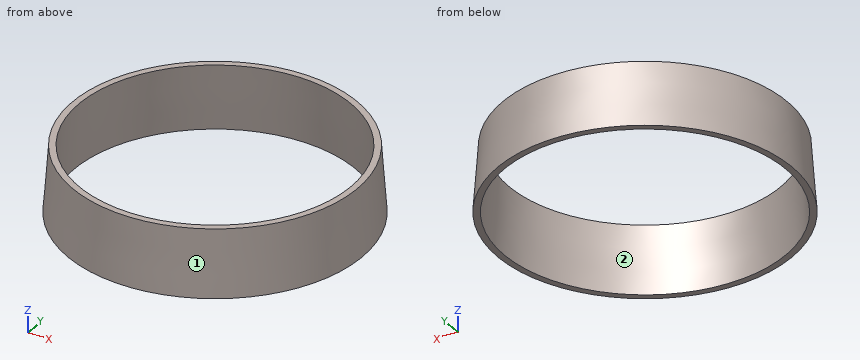
from build123d import *


with BuildPart() as cone_chico002:
    # Cone004 → Cone004 (revolve)
    with BuildSketch(Plane.XZ):
        Polygon((0, 0), (43.6, 0), (42.1, 20.5), (0, 20.5), align=None)
    revolve(axis=Axis((0, 0, 0), (0, 0, 1)))


with BuildPart() as cono001:
    # Cone005 → Cone005 (revolve)
    with BuildSketch(Plane.XZ):
        Polygon((0, 0), (45.6, 0), (44.1, 20.5), (0, 20.5), align=None)
    revolve(axis=Axis((0, 0, 0), (0, 0, 1)))

    # Cut015023: cut Cone_chico002
    add(cone_chico002.part, mode=Mode.SUBTRACT)


solid = cono001.part
Here's how the part is built. I have some questions about the finished solid (model axes, mm). Face numbers are marked on the shaded views. Round coordinates to 2 decimals unless told otherwise and drop trailing zeros. Order: outer loops, then holes, each group sorted by start corner. A loop starts at its lowest first (then second) coordinate and runs counter-clockwise, first axis right, second up. Notation, with made-up numbers: M 89,-10.5 L 117,-10.5 A24 ccw 117,6.5 Z; hole C 62,9.25 d8. An arc over 180 degrees is marked long. One line per question, with ' | ' between items.
1) Imagine slicing it at C-C, the plane z = 5.75. Write out the boundary of the cut face in (x, y).
Checked values:
outline: C 0,0 d90.36; hole C 0,0 d86.36
2) I need wall thicknesses on line 1 (X direction, y = 34.5, z = 13.75); line 2 (Y direction, x = 14.5, z = 5.5); line 3 (Y direction, x = 5.5, z = 5.25). Which ranges of each line are inside material? Lowest first, please.
Checked values:
line 1: x = -28.26 to -24.98, 24.98 to 28.26 | line 2: y = -42.81 to -40.69, 40.69 to 42.81 | line 3: y = -44.88 to -42.86, 42.86 to 44.88
3) We'd pull the mould along Y, two halves only. Please class the marked faces 1 and 2: released by +Y, released by -Y, zero draft, split by the parting line, or undercut.
Checked values:
face 1: split by the parting line | face 2: undercut
4) I'm going to push flat-ended pins straight in: pin 1 Ø2 at (y, z) = (-20, 13) entering from -X; pin 2 Ø3 at (x, z) = (-2.5, 15) entering from +Y; pin 3 Ø5 at (x, z) = (16, 4) entering from +Y. Where does each tip first touch, or does it pass through?
Checked values:
pin 1: stops at x = -40.41 | pin 2: stops at y = 44.56 | pin 3: stops at y = 43.27
5) Imagine slicing it at D-D, the plane z = 11. Write out the boundary of the cut face in (x, y), plus the area to 3 significant figures.
Checked values:
outline: C 0,0 d89.59; hole C 0,0 d85.59 | area: 550 mm²
